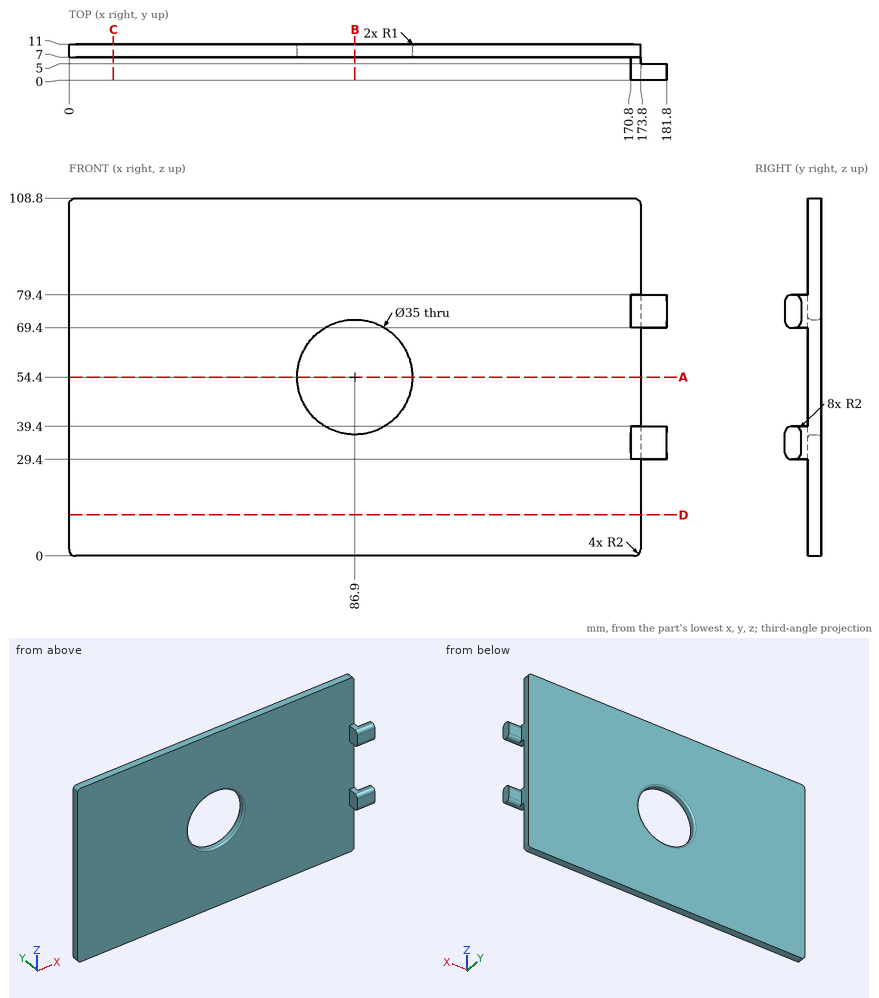
Can you work these out from the drawing? Everything is in mm from the part's minimum corner. Round coordinates to 2 decimals unless told otherwise and drop trailing zeros. Write each loop counter-clockwise with the first axis right and the second up, starting at its lowest first coordinate (ties: lowest second). Pieces come first, ordered by that corner, then holes. Notation, with made-up numbers: (21.25, 76.25) - (60.25, 76.25) arc R14 ccw to (60.25, 103.25) - close; hole circle Ø7 at (-1, 88). An arc over 180 degrees is marked (long way). Put each result on its own line as item: value. Start each with the question number.
(1) I want a section at C-C, the plane x = 13.5. Please give me the cut outline in (y, z), plus the area to 3 significant figures.
(2) I want a section at A-A, the plane z = 54.4. Please give me the cut outline in (x, y).
(3) Will these pins go through, and if not, where does the flat tip stop? pin 1 (6 mm diameter, centred on x = 59, z = 16, fed in from -Y); pin 2 (5 mm diameter, centred on y = 5.5, z = 74.5, fed in from -X); pin 3 (1.5 mm diameter, centred on x = 179, y = 4, fed in from +Z); pin 4 (5 mm diameter, centred on x = 176.5, z = 75.5, fed in from +Y).
(4) I want a section at B-B, the plane x = 86.9. Please give me the cut outline in (y, z), plus the area to 3 significant figures.
(5) I want a section at D-D, the plane z = 12.5. Please give me the cut outline in (x, y), plus the area to 3 significant figures.
(6) I need wall thicknesses on probe 1 along X at (y, z) = (9.2, 54.4); probe 2 along Z at (x, y) = (86.9, 8.65); probe 3 along Y at (x, z) = (142, 103). Which ranges of each line are inside material? Lowest first, please.
Here are the results:
1. outline: (7, 0) - (11, 0) - (11, 108.8) - (7, 108.8) - close
1. area: 435 mm^2
2. outline: (0, 7) - (68.4, 7) arc R1 ccw to (69.4, 8) - (69.4, 10) arc R1 ccw to (68.4, 11) - (0, 11) - close; (104.4, 8) arc R1 ccw to (105.4, 7) - (173.8, 7) - (173.8, 11) - (105.4, 11) arc R1 ccw to (104.4, 10) - close
3. pin 1: stops at y = 7
3. pin 2: stops at x = 0
3. pin 3: stops at z = 79.38
3. pin 4: stops at y = 5
4. outline: (7, 0) - (11, 0) - (11, 35.9) arc R1 ccw to (10, 36.9) - (8, 36.9) arc R1 ccw to (7, 35.9) - close; (7, 72.9) arc R1 ccw to (8, 71.9) - (10, 71.9) arc R1 ccw to (11, 72.9) - (11, 108.8) - (7, 108.8) - close
4. area: 294 mm^2
5. outline: (0, 7) - (173.8, 7) - (173.8, 11) - (0, 11) - close
5. area: 695 mm^2
6. probe 1: x = 0 to 69.4, 104.4 to 173.8
6. probe 2: z = 0 to 36.9, 71.9 to 108.8
6. probe 3: y = 7 to 11
